CAD build for the part. Positions are in the model's coordinates, mm. A direction names the side the tool comes from. Round coordinates to 2 decimals unless told otherwise and drop trailing zeros. Write each loop counter-clockwise with the first axis right and the second up, starting at its lowest first coordinate (ties: lowest second). Pieces come first, ordered by that corner, then holes. Notation, with made-up numbers: (79, 40.5) - (106, 40.5) arc R26 cw to (106, 60.5) - close; hole circle Ø8 at (-3, 53.5). An arc over 180 degrees is marked (long way). Put each result on its own line as item: value. Start each with the question number.
Item 1: Drill centre lines: line 1 (X direction, y = -6.5, z = -3.25); line 2 (Y direction, x = 5.7, z = 0); line 3 (Y direction, x = 2.35, z = 0). Where is each one in solid material? Low to high. Write a range as from..to.
Item 2: Mould opens along X. For faces 4 (the flat face through (0.935, -4, -6)), 5 (the flat face through (1.935, 8, 8)), 6 (the cylindrical face through (3.4, -11.4, 1.5)) say: released by +X, released by -X, zero draft, split by the parting line, or undercut.
Item 3: 3-axis set-ups, long thin cutter, end or side, ignore diameter. For faces 1 (the flat face through (0.985, -8.4, 0.8)), 2 (the cylindrical face through (3.45, 6.21, -3.23)), 3 (the cylindrical face through (4.682, 10.446, 2.32)): which of +Z, -Z, +X, -X, +Y, -Y reach the whole face in a straight line?
Item 4: Pin check, flat tips, straight feed: pin 1 Ø1.5 at (x, y) = (2, 9) entering from +Z; pin 2 Ø1.5 at (x, z) = (2.5, 2.5) entering from -Y; pin 3 Ø3 at (x, y) = (3, -2) entering from +Z. Stop position of each tip, or through.
Item 5: Cut at A-A (x = 5.55). Give the cut face in (y, z).
```python
from build123d import *

# Parameters (mm, degrees)
SMUSSO1_SIZE = 0.05


with BuildPart() as part:
    # Schizzo1 → Rivoluzione1 (revolve)
    with BuildSketch(Plane.XY, mode=Mode.PRIVATE) as rivoluzione1_sk:
        Polygon((0.935183111, 7), (1.935183111, 7), (1.935183111, 7.8), (2.435183111, 7.8), (2.435183111, 7), (4.435183111, 7), (4.435183111, 7.8), (4.935183111, 7.8), (4.935183111, 7), (5.935183111, 7), (5.935183111, 8.280172414), (5.885183111, 8.280172414), (5.885183111, 10.219827586), (5.935183111, 10.219827586), (5.935183111, 11.5), (4.935183111, 11.5), (4.935183111, 10.7), (4.435183111, 10.7), (4.435183111, 11.5), (2.435183111, 11.5), (2.435183111, 10.7), (1.935183111, 10.7), (1.935183111, 11.5), (0.935183111, 11.5), (0.935183111, 10.219827586), (0.985183111, 10.219827586), (0.985183111, 8.280172414), (0.935183111, 8.280172414), align=None)
    revolve(rivoluzione1_sk.sketch.rotate(Axis((0, 0, 0), (-1, 0, 0)), 90), axis=Axis((0, 0, 0), (-1, 0, 0)))

    # Smusso1
    smusso1_edges = [part.edges().sort_by_distance(p)[0] for p in [
        (0.935183111, 0, 8.280172414),
        (0.935183111, 0, 10.219827586),
        (0.935183111, 0, 11.5),
        (5.935183111, 0, 11.5),
        (5.935183111, 0, 10.219827586),
        (5.935183111, 0, 8.280172414),
        (5.935183111, 0, 7),
        (0.935183111, 0, 7),
    ]]
    chamfer(smusso1_edges, length=SMUSSO1_SIZE - 0.0001)  # a hair under: the kernel refuses the full size


solid = part.part
```
Output values:
1. line 1: 0.94..1.94, 2.44..4.44, 4.94..5.94
1. line 2: -11.5..-7, 7..11.5
1. line 3: -10.7..-7.8, 7.8..10.7
2. face 4: released by -X
2. face 5: undercut
2. face 6: zero draft
3. face 1: -X
3. face 2: +X, -X
3. face 3: none
4. pin 1: z = 8.01
4. pin 2: y = -11.37
4. pin 3: z = 11.49
5. outline: circle Ø23 at (0, 0); hole circle Ø14 at (0, 0)
